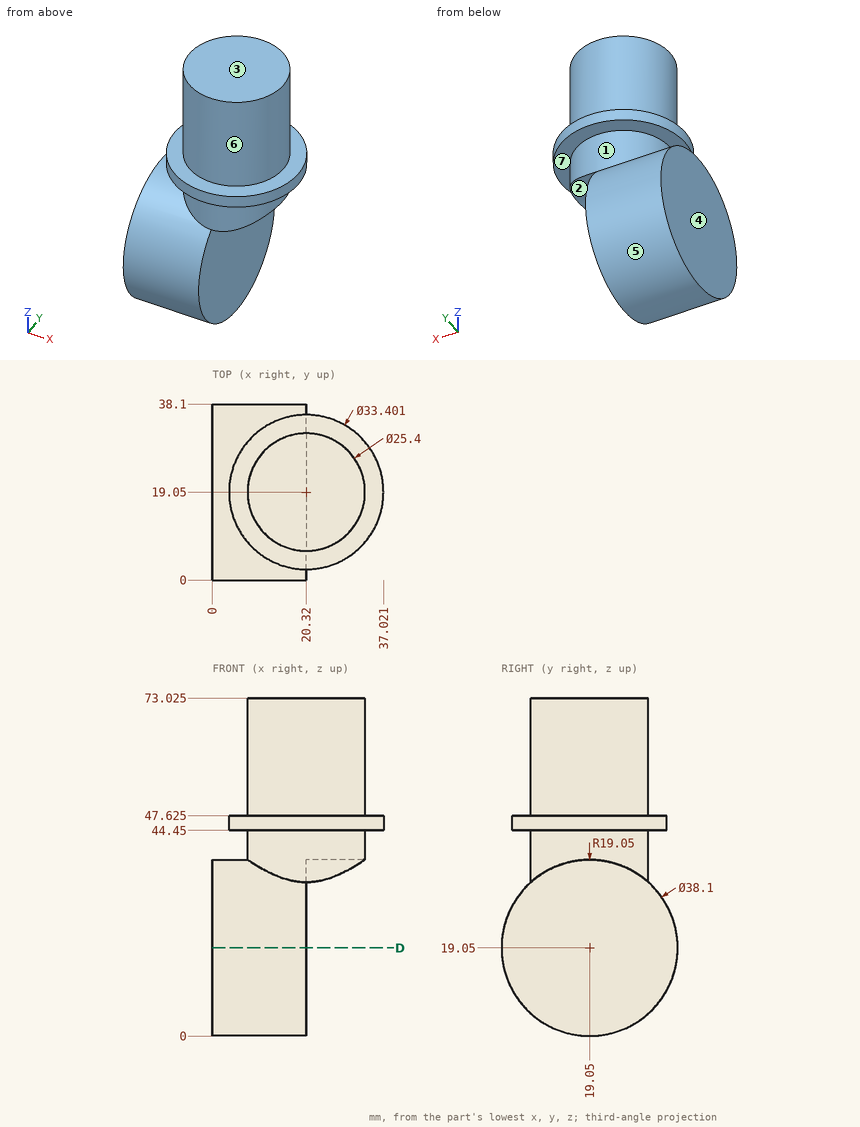
Check sheet for the drawn part. Datum: minimum x, y, z corner. Units: mm. A direction names the side the tool comes from. Coordinates: 2 decimals unless noted, no trailing zeros. Order: outer loops, then holes, each group sorted by start corner. A loop starts at its lowest first (then second) coordinate and runs counter-clockwise, first axis right, second up. Notation, with made-up numbers: (-17.75, -3) - (12.25, -3) arc R27 cw to (12.25, 34) - close; hole circle Ø2 at (2.5, -28.5). An arc over 180 degrees is marked (long way). Return JSON: item names as keys, results as strings.
(1) Thickness scan on line 1 along Y through (x, z) = (10.5, 18.5); line 2 along X through (y, z) = (20, 15); line 3 along Y through (x, z) = (14, 28) (1 decimal). Record the ranges inside material, lowest first.
Filled sheet:
{"line 1": "y = 0.01 to 38.09", "line 2": "x = 0 to 20.32", "line 3": "y = 2.2 to 35.9"}
(2) Access from +Z, -Z, +X, -X, +Y, -Y to the whole of each face (thin tool, end or side, straight path). Record for the marked faces 4, 5, 6 and 7.
Filled sheet:
{"face 4": "+Z, -Z, -X, +Y, -Y", "face 5": "-X", "face 6": "+Z", "face 7": "none"}
(3) Go/stop test with flat-tipped pins: pin 1 (6 mm diameter, centred on x = 32, z = 36.5, fed in from -Y); pin 2 (12 mm diameter, centred on y = 27, z = 37.5, fed in from +X); pin 3 (2 mm diameter, centred on x = 25.5, z = 38.5, fed in from +Y). Record where each tip stops, or that it passes through.
Filled sheet:
{"pin 1": "stops at y = 9.78", "pin 2": "stops at x = 32.87", "pin 3": "stops at y = 31.04"}
(4) Section check D-D, the plane z = 19.05. Record the cut outline in (x, y), and give its area (3 significant figures).
Filled sheet:
{"outline": "(0, 0) - (20.32, 0) - (20.32, 38.1) - (0, 38.1) - close", "area": "774 mm^2"}
(5) Mould release check, pull along Y, two halves, no side actions. Record for the marked faces 1, 2 and 3: pulls with the +Y half, pulls with the -Y half, needs draft (parallel to the pull), parting line crosses it, or undercut.
Filled sheet:
{"face 1": "parting line crosses it", "face 2": "undercut", "face 3": "needs draft"}
